Design review of the part shown in the three views and the two pictorial views. Dimensions are in mm from the part's minimum x, y and z. A direction names the side the tool comes from. Round coordinates to 2 decimals unless told otherwise and drop trailing zeros. Order: outer loops, then holes, each group sorted by start corner. A loop starts at its lowest first (then second) coordinate and runs counter-clockwise, first axis right, second up. Notation, with made-up numbers: M 31,10 L 88,10 A28 ccw 88,32 Z; hole C 89,88.5 d3. An arc over 180 degrees is marked long. Write item = value, one per line. Start each with the question number.
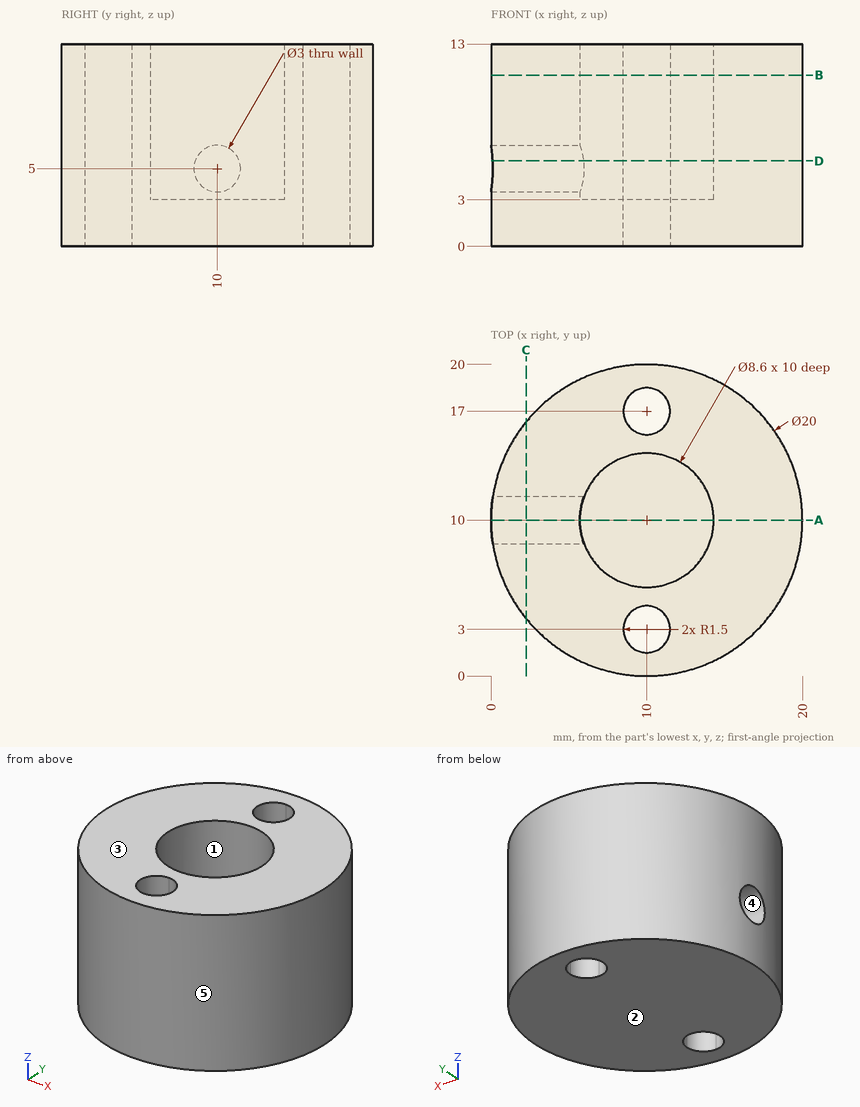
(1) For line 1 along Y through (x, z) = (9.5, 2.75); line 2 along X through (y, z) = (11.5, 7.5); line 3 along Y through (x, z) = (6.25, 8.5), list the stretches that pass through material, from the lowest coordinate up.
(2) We need section B-B, the plane z = 11. Write out the cut boundary in (x, y), then the cut area to 3 significant figures.
(3) We need section D-D, the plane z = 5.5. Write out the cut boundary in (x, y), then the cut area to 3 significant figures.
(4) We need section C-C, the plane x = 2.25. Write out the cut boundary in (y, z).
(5) We need section A-A, the plane y = 10. Write out the cut boundary in (x, z), then the cut area to 3 significant figures.
(6) Insertion check: pin 1 (1 mm diameter, centred on y = 2, z = 9, fed in from -X); pin 2 (1 mm diameter, centred on y = 15.5, z = 4, fed in from -X); pin 3 (6 mm diameter, centred on y = 5, z = 2, fed in from -X). Each pin has a flat end and moves straight along its axis. Give the tip position at first contact, or say it passes through.
(7) For the marked faces 1 and 2, list the 3-axis set-ups (+Z, -Z, +X, -X, +Y, -Y) from which the entire face can be reached by the end or side of a thin tool; tool diameter is ignored.
(8) Draft analysis for pull direction Y (two halves, no side actions). For the marked faces 3, 4 and 5, state which applies: released by +Y, released by -Y, zero draft, split by the parting line, or undercut.
Values:
q1.line_1 = 0.01 to 1.59, 4.41 to 15.59, 18.41 to 19.99
q1.line_2 = 0.11 to 5.97, 14.03 to 19.89
q1.line_3 = 0.73 to 7.9, 12.1 to 19.27
q2.outline = C 10,10 d20; hole C 10,10 d8.6; hole M 10,4.5 A1.5 ccw long 11.5,3 A1.5 ccw Z; hole M 10,18.5 A1.5 ccw long 11.5,17 A1.5 ccw Z
q2.area = 242 mm²
q3.outline = M 0.1,8.59 A10 ccw long 0.1,11.41 L 5.94,11.41 A4.3 cw long 5.94,8.59 Z; hole M 10,4.5 A1.5 ccw long 11.5,3 A1.5 ccw Z; hole M 10,18.5 A1.5 ccw long 11.5,17 A1.5 ccw Z
q3.area = 226 mm²
q4.outline = M 3.68,0 L 16.32,0 L 16.32,13 L 3.68,13 Z; hole C 10,5 d3
q5.outline = M 0,0 L 20,0 L 20,13 L 14.3,13 L 14.3,3 L 5.7,3 L 5.7,3.5 L 0,3.5 Z; M 0,6.5 L 5.7,6.5 L 5.7,13 L 0,13 Z
q5.area = 157 mm²
q6.pin_1 = 3.39
q6.pin_2 = 1.34
q6.pin_3 = 0.2
q7.face_1 = +Z
q7.face_2 = -Z, +X, -X, +Y, -Y
q8.face_3 = zero draft
q8.face_4 = undercut
q8.face_5 = split by the parting line
